from build123d import *

# Parameters (mm, degrees)
BOSS_EXTRUDE1_DEPTH = 25
CUT_EXTRUDE1_DEPTH  = 44.301270189
SKETCH3_R           = 1.75
CUT_EXTRUDE2_DEPTH  = 42.641325627


with BuildPart() as part:
    # Sketch1 → Boss-Extrude1 (new body)
    with BuildSketch(Plane(origin=(0, 0, 0), x_dir=(0, 0, -1), z_dir=(1, 0, 0))):
        with BuildLine():
            Line((-25, 0), (-25, 3))
            Line((-25, 3), (-15.2, 3))
            Line((-15.2, 3), (-15.2, 9.8))
            ThreePointArc((-15.2, 9.8), (0, 25), (15.2, 9.8))
            Line((15.2, 9.8), (15.2, 3))
            Line((15.2, 3), (25, 3))
            Line((25, 3), (25, 0))
            Line((25, 0), (-25, 0))
        make_face()
    extrude(amount=BOSS_EXTRUDE1_DEPTH)

    # Sketch2 → Cut-Extrude1 (cut, through all)
    with BuildSketch(Plane(origin=(25, 0, 0), x_dir=(0, 0, -1), z_dir=(1, 0, 0))):
        with BuildLine():
            Line((-12, 10), (-12, 0))
            Line((-12, 0), (12, 0))
            Line((12, 0), (12, 10))
            ThreePointArc((12, 10), (0, 22), (-12, 10))
        make_face()
    extrude(amount=-CUT_EXTRUDE1_DEPTH, mode=Mode.SUBTRACT)

    # Sketch3 → Cut-Extrude2 (cut, through all)
    with BuildSketch(Plane(origin=(0, 3, 0), x_dir=(1, 0, 0), z_dir=(0, 1, 0))):
        with Locations(Location((5, -20, 0), (0, 0, 270))):
            Circle(SKETCH3_R)
        with Locations(Location((20, -20, 0), (0, 0, 270))):
            Circle(SKETCH3_R)
        with Locations(Location((5, 20, 0), (0, 0, 270))):
            Circle(SKETCH3_R)
        with Locations(Location((20, 20, 0), (0, 0, 270))):
            Circle(SKETCH3_R)
    extrude(amount=-CUT_EXTRUDE2_DEPTH, mode=Mode.SUBTRACT)


solid = part.part
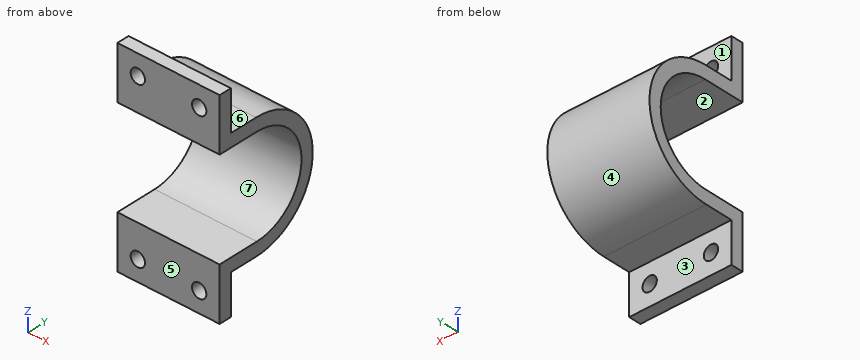
Work out the finished part from the listing and answer in its coordinate system (mm). Face numbers are marked on the shaded views. A direction names the side the tool comes from. Give positions to 0.01 mm unless a question says otherwise; leave off trailing zeros. Loops run counter-clockwise (first coordinate to the right, second up) from the corner with the lowest first, then second, coordinate; pieces in that order, holes last. Notation, with made-up numbers: (75.5, 75) - (103.5, 75) arc R18 cw to (103.5, 110) - close; hole circle Ø2 at (47.5, 3.5). An arc over 180 degrees is marked (long way). Answer in a Markdown table with one row per item.
(1) For a pull along Z with two mould halves and no side action, classify the marked faces 5, 6 and 7 as pulls with the +Z half, pulls with the -Z half, needs draft (parallel to the pull), parting line crosses it, or undercut.
Results list:
| item | result |
|---|---|
| face 5 | needs draft |
| face 6 | pulls with the +Z half |
| face 7 | undercut |
(2) Section A-A (z = 20) is taken. Give the vertices of the cut face in (x, y).
Results list:
| item | result |
|---|---|
| outline | (0, 0) - (3.25, 0) - (3.25, 3) - (0, 3) - close; (6.75, 0) - (18.25, 0) - (18.25, 3) - (6.75, 3) - close; (21.75, 0) - (25, 0) - (25, 3) - (21.75, 3) - close |
(3) Section B-B (x = 20) is taken. Give the vertices of the cut face in (y, z), and give its area (3 significant figures).
Results list:
| item | result |
|---|---|
| outline | (0, -25) - (3, -25) - (3, -21.75) - (0, -21.75) - close; (0, -18.25) - (3, -18.25) - (3, -15.2) - (9.8, -15.2) arc R15.2 ccw to (9.8, 15.2) - (3, 15.2) - (3, 18.25) - (0, 18.25) - (0, 12) - (10, 12) arc R12 cw to (10, -12) - (0, -12) - close; (0, 21.75) - (3, 21.75) - (3, 25) - (0, 25) - close |
| area | 232 mm² |
(4) A tool of negligible diameter and unlimited length cuts with its end or side. For the marked faces 1, 2, 3 and 4, from which of +Z, -Z, +X, -X, +Y, -Y can it reach the whole face along a straight path? Write none if from no direction.
Results list:
| item | result |
|---|---|
| face 1 | +Z, +X, -X, +Y |
| face 2 | +X, -X, -Y |
| face 3 | -Z, +X, -X, +Y |
| face 4 | +X, -X, +Y |
(5) Section D-D (x = 12.75) is taken. Give the vertices of the cut face in (y, z), and give its area (3 significant figures).
Results list:
| item | result |
|---|---|
| outline | (0, -25) - (3, -25) - (3, -15.2) - (9.8, -15.2) arc R15.2 ccw to (9.8, 15.2) - (3, 15.2) - (3, 25) - (0, 25) - (0, 12) - (10, 12) arc R12 cw to (10, -12) - (0, -12) - close |
| area | 253 mm² |
(6) Section C-C (y = 21.25) is taken. Give the vertices of the cut face in (x, z).
Results list:
| item | result |
|---|---|
| outline | (0, -10) - (25, -10) - (25, -4.18) - (0, -4.18) - close; (0, 4.18) - (25, 4.18) - (25, 10) - (0, 10) - close |
(7) Flat-ended cylindrical pins translate along their axes: pin 1 Ø4 at (x, y) = (19, 13.5) entering from +Z; pin 2 Ø3 at (x, z) = (5, -20) entering from +Y; pin 3 Ø6 at (x, z) = (16, -6.5) entering from +Y; pin 4 Ø2 at (x, y) = (17, 18.5) entering from -Z. Find the tip coordinate at first contact, or state that the pin passes through.
Results list:
| item | result |
|---|---|
| pin 1 | stops at z = 15.1 |
| pin 2 | passes through |
| pin 3 | stops at y = 24.59 |
| pin 4 | stops at z = -13.11 |
(8) Consider L1, parallel to X at y = 1.25, z = 20; L2, parallel to Z at x = 17.25, y = 10.25; L3, parallel to Z at x = 24.25, y = 19.25. Determine where each line is inside the solid, lowest interval first. Write a range as [from, to].
Results list:
| item | result |
|---|---|
| L1 | x = [0, 3.25], [6.75, 18.25], [21.75, 25] |
| L2 | z = [-15.19, -12], [12, 15.19] |
| L3 | z = [-11.91, -7.64], [7.64, 11.91] |
